Model file for the job. Use its own axes, mm. A direction names the side the tool comes from. Give positions to 0.01 mm unless a question says otherwise; leave off trailing zeros. Write each loop counter-clockwise with the first axis right and the second up, starting at its lowest first coordinate (ties: lowest second). Pieces come first, ordered by that corner, then holes. Notation, with made-up numbers: (-15, 68) - (44, 68) arc R12 ccw to (44, 83) - close; hole circle Ø10 at (18.5, -30.75). An arc over 180 degrees is marked (long way). One line per item, written item: value. Start each with the question number.
(1) Cut at C-C, the plane y = -109.5. List the corners of the cut face in (x, z), and give its area (3 significant figures).
(2) Cut at D-D, the plane x = 25.5. List the corners of the cut face in (y, z).
(3) Probe L1, parallel to Z at x = -33, y = -48; L2, parallel to Y at x = -8, z = -32; L3, parallel to Y at x = -38.5, z = 35. List the from-to ranges inside material, lowest first.
(4) 3-axis set-ups, long thin cutter, end or side, ignore diameter. For faces 1 (the face through (34, -92.606, 50)), 2 (the face through (17.06, -100, 50)), 3 (the face through (-50.171, -116, 29)): which of +Z, -Z, +X, -X, +Y, -Y reach the whole face in a straight line?
(5) Cut at B-B, the plane z = 0. List the corners of the cut face in (x, y).
(6) Cut at A-A, the plane x = 0. List the corners of the cut face in (y, z), and give its area (3 significant figures).
(7) Mould opens along X. For faces 4 (the face through (-28.109, -116, 29)), 5 (the face through (-56.709, -56, -1)), 6 (the face through (-1, -56, 45.293)) say: pulls with the +X half, pulls with the -X half, needs draft (parallel to the pull), parting line crosses it, or undercut.
(8) Drop flat-ended pins along their axis: P1, Ø1.5, axis at x = 44, z = 22.5, coming from the +Y side; P2, Ø2.5, axis at x = -34, y = -115.5, coming from the -Z side; P3, Ø3, axis at x = 32.5, z = 50, coming from the -Y side; P4, Ø3, axis at y = -97, z = 49, coming from the +X side. Give the stop position or say it passes through.
from build123d import *

# Parameters (mm, degrees)
F0_W      = 113.6225089431
F0_H      = 91.5519557893
F1_DEPTH  = 113.62251
F2_R      = 28.629575464
F3_DEPTH  = 10
F4_DEPTH  = 18
F7_W      = 33.8436812162
F7_H      = 14.7902220488
F8_DEPTH  = 10
F9_W      = 22.0619104803
F9_H      = 14.1544528306
F10_DEPTH = 5
F11_W     = 113.6225089431
F11_H     = 91.5519557893
F12_DEPTH = 60


# Not quite as in the source:
# - the program builds the solid bodies; features that only make, move or delete a surface that nothing else refers to are left out


with BuildPart() as f1:
    # F0 (on Front) → F1 (new body)
    with BuildSketch(Plane.XZ):
        with Locations((0.1021772623, -0.4832614213)):
            Rectangle(F0_W, F0_H)
    extrude(amount=F1_DEPTH)

    # F2 (on face) → F3 (join)
    with BuildSketch(Plane.XZ.offset(113.62251)):
        Circle(F2_R)
    extrude(amount=F3_DEPTH)

    # F4 (add): a face of the model
    f4_faces = [f1.faces().sort_by_distance(p)[0] for p in [
        (0, -123.62251, 0),
    ]]
    extrude(f4_faces, amount=-F4_DEPTH)

    # F7 (on face) → F8 (join)
    with BuildSketch(Plane.XY.offset(45.2927164733)):
        with Locations((33.9821465313, -100.0008359551)):
            Rectangle(F7_W, F7_H)
    extrude(amount=F8_DEPTH)

    # F9 (on face) → F10 (join)
    with BuildSketch(Plane.XZ.offset(113.62251)):
        with Locations((-39.1396004707, 29.0038492531)):
            Rectangle(F9_W, F9_H)
    extrude(amount=F10_DEPTH)

    # F11 (on face) → F12 (join)
    with BuildSketch(Plane(origin=(0, 0, 0), x_dir=(-1, 0, 0), z_dir=(0, 1, 0))):
        with Locations((-0.1021772623, -0.4832614213)):
            Rectangle(F11_W, F11_H)
    extrude(amount=-F12_DEPTH)


solid = f1.part
Answers follow:
1. outline: (-56.71, -46.26) - (56.91, -46.26) - (56.91, 45.29) - (-56.71, 45.29) - close
1. area: 10,400 mm²
2. outline: (-123.62, -13.02) - (-113.62, -13.02) - (-113.62, -46.26) - (0, -46.26) - (0, 45.29) - (-92.61, 45.29) - (-92.61, 55.29) - (-107.4, 55.29) - (-107.4, 45.29) - (-113.62, 45.29) - (-113.62, 13.02) - (-123.62, 13.02) - close
3. L1: z = -46.26 to 45.29
3. L2: y = -113.62 to 0
3. L3: y = -118.62 to 0
4. face 1: +Z, +X, -X, +Y
4. face 2: +Z, -X, +Y, -Y
4. face 3: +Z, -Z, -X, -Y
5. outline: (-56.71, -113.62) - (-28.63, -113.62) - (-28.63, -123.62) - (28.63, -123.62) - (28.63, -113.62) - (56.91, -113.62) - (56.91, 0) - (-56.71, 0) - close
6. outline: (-123.62, -28.63) - (-113.62, -28.63) - (-113.62, -46.26) - (0, -46.26) - (0, 45.29) - (-113.62, 45.29) - (-113.62, 28.63) - (-123.62, 28.63) - close
6. area: 11,000 mm²
7. face 4: undercut
7. face 5: pulls with the -X half
7. face 6: needs draft
8. P1: stops at y = 0
8. P2: stops at z = 21.93
8. P3: stops at y = -107.4
8. P4: stops at x = 50.9
